from build123d import *

# Parameters (mm, degrees)
SKETCH1_W           = 19
SKETCH1_H           = 40
BOSS_EXTRUDE1_DEPTH = 2
SKETCH2_W           = 19
SKETCH2_H           = 2
BOSS_EXTRUDE2_DEPTH = 38
SKETCH3_R           = 2
CUT_EXTRUDE1_DEPTH  = 10
SKETCH4_R           = 2
CUT_EXTRUDE2_DEPTH  = 10


with BuildPart() as part:
    # Sketch1 → Boss-Extrude1 (new body)
    with BuildSketch(Plane.XY):
        Rectangle(SKETCH1_W, SKETCH1_H)
    extrude(amount=BOSS_EXTRUDE1_DEPTH)

    # Sketch2 → Boss-Extrude2 (add)
    with BuildSketch(Plane.XY.offset(2)):
        with Locations((0, 19)):
            Rectangle(SKETCH2_W, SKETCH2_H)
    extrude(amount=BOSS_EXTRUDE2_DEPTH)

    # Sketch3 → Cut-Extrude1 (cut)
    with BuildSketch(Plane(origin=(0, 0, 0), x_dir=(-1, 0, 0), z_dir=(0, 0, -1))):
        with Locations((0, 10)):
            Circle(SKETCH3_R)
        with Locations((0, -10)):
            Circle(SKETCH3_R)
    extrude(amount=-CUT_EXTRUDE1_DEPTH, mode=Mode.SUBTRACT)

    # Sketch4 → Cut-Extrude2 (cut)
    with BuildSketch(Plane(origin=(0, 20, 0), x_dir=(1, 0, 0), z_dir=(0, 1, 0))):
        with Locations(Location((0, -10, 0), (0, 0, 270))):
            Circle(SKETCH4_R)
        with Locations(Location((0, -30, 0), (0, 0, 270))):
            Circle(SKETCH4_R)
    extrude(amount=-CUT_EXTRUDE2_DEPTH, mode=Mode.SUBTRACT)


solid = part.part
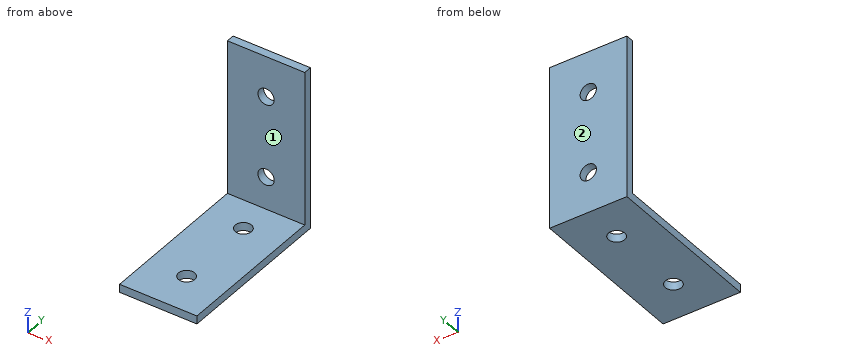
Part model, mm, in its own coordinate system. Face numbers are marked on the shaded views. A direction names the side the tool comes from. Coordinates: 2 decimals unless noted, no trailing zeros. Order: outer loops, then holes, each group sorted by start corner. A loop starts at its lowest first (then second) coordinate and runs counter-clockwise, first axis right, second up. Notation, with made-up numbers: M -36.75,56.5 L -23.75,56.5 A34 cw -23.75,88.5 Z; hole C 67.25,36.25 d11. An arc over 180 degrees is marked long. One line per question, with ' | ' between items.
Q1. Slice it at D-D (x = 3). Give the cut face in (y, z), and give its area (3 significant figures).
A:
outline: M -20,0 L 20,0 L 20,40 L 18,40 L 18,2 L -20,2 Z | area: 156 mm^2
Q2. Slice it at C-C (z = 10). Give the cut face in (x, y), and give its area (3 significant figures).
A:
outline: M -9.5,18 L -2,18 L -2,20 L -9.5,20 Z; M 2,18 L 9.5,18 L 9.5,20 L 2,20 Z | area: 30.0 mm^2
Q3. Slice it at B-B (x = 0). Give the cut face in (y, z).
A:
outline: M -20,0 L -12,0 L -12,2 L -20,2 Z; M -8,0 L 8,0 L 8,2 L -8,2 Z; M 12,0 L 20,0 L 20,8 L 18,8 L 18,2 L 12,2 Z; M 18,12 L 20,12 L 20,28 L 18,28 Z; M 18,32 L 20,32 L 20,40 L 18,40 Z
Q4. 3-axis set-ups, long thin cutter, end or side, ignore diameter. For the marked faces 1 and 2: which of +Z, -Z, +X, -X, +Y, -Y reach the whole face in a straight line?
A:
face 1: +Z, +X, -X, -Y | face 2: +Z, -Z, +X, -X, +Y
Q5. Slice it at A-A (y = 10). Give the cut face in (x, z).
A:
outline: M -9.5,0 L -2,0 L -2,2 L -9.5,2 Z; M 2,0 L 9.5,0 L 9.5,2 L 2,2 Z
Q6. Drill centre lines: line 1 (Y direction, x = 0, z = 0.4); line 2 (X direction, y = 19.55, z = 10); line 3 (Z direction, x = 8.5, y = -17.5). Where is each one in solid material? Low to high.
A:
line 1: y = -20 to -12, -8 to 8, 12 to 20 | line 2: x = -9.5 to -2, 2 to 9.5 | line 3: z = 0 to 2
Q7. Pin check, flat tips, straight feed: P1, Ø2.5, axis at x = 0, z = 10, coming from the +Y side; P2, Ø1, axis at x = 7, z = 12, coming from the -Y side; P3, Ø5.5, axis at x = -2, y = 2, coming from the +Z side. Stop position of each tip, or through.
A:
P1: passes through | P2: stops at y = 18 | P3: stops at z = 2
